```python
from build123d import *

# Parameters (mm, degrees)
SKETCH1_R                   = 49.25
MAINTUBE_DEPTH              = 1239
SKETCH2_R                   = 50.45
NOZZLERETAINER_DEPTH        = 13
SKETCH3_R                   = 23.75
MOUNTSHOULDER_DEPTH         = 31
SKETCH4_R                   = 11.125
MOUNTNECK_DEPTH             = 27.2
F_3_8_16_TAPPED_HOLE1_D     = 7.9375
F_3_8_16_TAPPED_HOLE1_DEPTH = 27.3
F_3_8_16_TAPPED_HOLE1_TIP   = 2.384665582


with BuildPart() as part:
    # Sketch1 → mainTube (new body)
    with BuildSketch(Plane(origin=(0, 0, 0), x_dir=(1, 0, 0), z_dir=(0, 1, 0))):
        with Locations(Location((0, 0, 0), (0, 0, 270))):
            Circle(SKETCH1_R)
    extrude(amount=MAINTUBE_DEPTH)

    # Sketch2 → nozzleRetainer (add)
    with BuildSketch(Plane.XZ):
        with Locations(Location((0, 0, 0), (0, 0, 90))):
            Circle(SKETCH2_R)
    extrude(amount=NOZZLERETAINER_DEPTH)

    # Sketch3 → mountShoulder (add)
    with BuildSketch(Plane(origin=(0, 1239, 0), x_dir=(1, 0, 0), z_dir=(0, 1, 0))):
        with Locations(Location((0, 0, 0), (0, 0, 270))):
            Circle(SKETCH3_R)
    extrude(amount=MOUNTSHOULDER_DEPTH)

    # Sketch4 → mountNeck (add)
    with BuildSketch(Plane(origin=(0, 1270, 0), x_dir=(1, 0, 0), z_dir=(0, 1, 0))):
        with Locations(Location((0, 0, 0), (0, 0, 270))):
            Circle(SKETCH4_R)
    extrude(amount=MOUNTNECK_DEPTH)

    # 3/8-16 Tapped Hole1
    with Locations(Plane(origin=(0, 1297.2, 0), x_dir=(1, 0, 0), z_dir=(0, 1, 0))):
        with Locations((0, 0)):
            Hole(F_3_8_16_TAPPED_HOLE1_D / 2, depth=F_3_8_16_TAPPED_HOLE1_DEPTH)
            with Locations((0, 0, -(F_3_8_16_TAPPED_HOLE1_DEPTH + F_3_8_16_TAPPED_HOLE1_TIP / 2))):  # 118° drill point
                Cone(0, F_3_8_16_TAPPED_HOLE1_D / 2, F_3_8_16_TAPPED_HOLE1_TIP, mode=Mode.SUBTRACT)


solid = part.part
```
CAD build for the part. Positions are in the model's coordinates, mm. A direction names the side the tool comes from. Give positions to 0.01 mm unless a question says otherwise; leave off trailing zeros. Order: outer loops, then holes, each group sorted by start corner. A loop starts at its lowest first (then second) coordinate and runs counter-clockwise, first axis right, second up. Notation, with made-up numbers: M 18,14 L 69,14 A28 cw 69,47 Z; hole C -3,65.25 d7. An arc over 180 degrees is marked long. Put each result on its own line as item: value. Start each with the question number.
(1) Saw through at A-A, the plane z = -36. Write the cut outline in (x, y), then the cut area to 3 significant figures.
(2) Saw through at B-B, the plane y = 408.5. Write the cut outline in (x, z).
(3) Flat gauge pins, fed straight in: pin 1 Ø5 at (x, z) = (1, 39) entering from +Y; pin 2 Ø10 at (y, z) = (759.5, -34) entering from +X; pin 3 Ø4 at (x, y) = (29, 588) entering from +Z. Where does each tip first touch, or does it go through?
(4) Which spindle directions (+Z, -Z, +X, -X, +Y, -Y) get a long thin tool onto all of the face, cutting with end or side? Do faces 1 (the flat face through (-1, -13, -1)), 2 (the flat face through (48.3, 0, 11)). Say none if no direction does.
(5) Saw through at C-C, the plane x = 35.5. Write the cut outline in (y, z).
(6) Drill centre lines: line 1 along X through (y, z) = (889, 0); line 2 along Y through (x, z) = (20.5, -21); line 3 along Y through (x, z) = (-28, 41). Where is each one in solid material? Low to high.
Check result:
1. outline: M -35.34,-13 L 35.34,-13 L 35.34,0 L 33.61,0 L 33.61,1239 L -33.61,1239 L -33.61,0 L -35.34,0 Z
1. area: 84,200 mm2
2. outline: C 0,0 d98.5
3. pin 1: stops at y = 1239
3. pin 2: stops at x = 39.81
3. pin 3: stops at z = 41.19
4. face 1: +Z, -Z, +X, -X, -Y
4. face 2: +Y
5. outline: M -13,-35.85 L 0,-35.85 L 0,-34.14 L 1239,-34.14 L 1239,34.14 L 0,34.14 L 0,35.85 L -13,35.85 Z
6. line 1: x = -49.25 to 49.25
6. line 2: y = -13 to 1239
6. line 3: y = -13 to 0
